Geometry check sheet. Reference: the model listing, model coordinates, mm. A direction names the side the tool comes from. Give positions to 0.01 mm unless a question says otherwise; leave off trailing zeros. Loops run counter-clockwise (first coordinate to the right, second up) from the corner with the lowest first, then second, coordinate; pieces in that order, holes last.
```python
from build123d import *

# Parameters (mm, degrees)
SKETCH1_R           = 60.5
SKETCH1_R_2         = 2.5
BOSS_EXTRUDE1_DEPTH = 5
SKETCH2_R           = 5
CUT_EXTRUDE1_DEPTH  = 2
SKETCH4_R           = 2
CUT_EXTRUDE2_DEPTH  = 86.612499087


with BuildPart() as part:
    # Sketch1 → Boss-Extrude1 (new body)
    with BuildSketch(Plane(origin=(0, 0, 0), x_dir=(1, 0, 0), z_dir=(0, 1, 0))):
        with Locations(Location((0, 0, 0), (0, 0, 270))):
            Circle(SKETCH1_R)
        with Locations(Location((0, 0, 0), (0, 0, 270))):
            Circle(SKETCH1_R_2, mode=Mode.SUBTRACT)
    extrude(amount=BOSS_EXTRUDE1_DEPTH)

    # Sketch2 → Cut-Extrude1 (cut)
    with BuildSketch(Plane.XZ):
        with Locations(Location((0, 53, 0), (0, 0, 270))):
            Circle(SKETCH2_R)
        with Locations(Location((53, 0, 0), (0, 0, 270))):
            Circle(SKETCH2_R)
        with Locations(Location((0, -53, 0), (0, 0, 270))):
            Circle(SKETCH2_R)
        with Locations(Location((-53, 0, 0), (0, 0, 270))):
            Circle(SKETCH2_R)
    extrude(amount=-CUT_EXTRUDE1_DEPTH, mode=Mode.SUBTRACT)

    # Sketch4 → Cut-Extrude2 (cut, through all)
    with BuildSketch(Plane(origin=(0, 2, 0), x_dir=(-1, 0, 0), z_dir=(0, -1, 0))):
        with Locations(Location((0, -53, 0), (0, 0, 90))):
            Circle(SKETCH4_R)
        with Locations(Location((-53, 0, 0), (0, 0, 90))):
            Circle(SKETCH4_R)
        with Locations(Location((0, 53, 0), (0, 0, 90))):
            Circle(SKETCH4_R)
        with Locations(Location((53, 0, 0), (0, 0, 90))):
            Circle(SKETCH4_R)
    extrude(amount=-CUT_EXTRUDE2_DEPTH, mode=Mode.SUBTRACT)


solid = part.part
```
1) Sectioned sample at B-B on x = 0. Enter the section's corners in (y, z).
2) Sectioned sample at C-C on y = 0.9. Enter the section's corners in (x, z), plus the area to 3 significant figures.
3) Sectioned sample at A-A on z = 0. Enter the section's corners in (x, y).
4) Tool access check on faces 4 (the cylindrical face through (0, 3, 55)), 5 (the flat face through (0.1, 2, -55.2)). Record the directions out of +Z, -Z, +X, -X, +Y, -Y that give a thin tool (end or side, any length) a straight path to the whole face; none if there is none.
5) Depth check by flat-ended pin: P1, Ø4.5, axis at x = -53, z = 0, coming from the -Y side; P2, Ø2, axis at x = 41.5, y = 1, coming from the -Z side; P3, Ø3, axis at x = 0, z = 0, coming from the -Y side; P4, Ø3, axis at x = -10.5, y = 4, coming from the -Z side. Enter the tip coordinate at first touch or a pass-through.
6) Scan lines: line 1 along X through (y, z) = (3.65, 0); line 2 along X through (y, z) = (0.95, 53); line 3 along X through (y, z) = (0.55, -54.5). Record each from-to range of solid material in increasing order.
7) Sectioned sample at D-D on z = 53. Enter the section's corners in (x, y).
8) Mould release check, pull along X, two halves, no side actions. Record for faces 1 (the flat face through (0.1, 2, 50.8)), 2 (the cylindrical face through (-59.06, 2.46, -13.12)), 3 (the flat face through (1, 5, 13)): +X half, -X half, draft (parallel to the pull), parting line (faces both ways), or undercut.
Determined:
1. outline: (0, -60.5) - (5, -60.5) - (5, -55) - (2, -55) - (2, -58) - (0, -58) - close; (0, -48) - (2, -48) - (2, -51) - (5, -51) - (5, -2.5) - (0, -2.5) - close; (0, 2.5) - (5, 2.5) - (5, 51) - (2, 51) - (2, 48) - (0, 48) - close; (0, 58) - (2, 58) - (2, 55) - (5, 55) - (5, 60.5) - (0, 60.5) - close
2. outline: circle Ø121 at (0, 0); hole circle Ø10 at (-53, 0); hole circle Ø10 at (0, -53); hole circle Ø10 at (0, 53); hole circle Ø5 at (0, 0); hole circle Ø10 at (53, 0)
2. area: 11,200 mm2
3. outline: (-60.5, 0) - (-58, 0) - (-58, 2) - (-55, 2) - (-55, 5) - (-60.5, 5) - close; (-51, 2) - (-48, 2) - (-48, 0) - (-2.5, 0) - (-2.5, 5) - (-51, 5) - close; (2.5, 0) - (48, 0) - (48, 2) - (51, 2) - (51, 5) - (2.5, 5) - close; (55, 2) - (58, 2) - (58, 0) - (60.5, 0) - (60.5, 5) - (55, 5) - close
4. face 4: +Y, -Y
4. face 5: -Y
5. P1: stops at y = 2
5. P2: stops at z = -44.94
5. P3: passes through
5. P4: stops at z = -59.83
6. line 1: x = -60.5 to -55, -51 to -2.5, 2.5 to 51, 55 to 60.5
6. line 2: x = -29.18 to -5, 5 to 29.18
6. line 3: x = -26.27 to -4.77, 4.77 to 26.27
7. outline: (-29.18, 0) - (-5, 0) - (-5, 2) - (-2, 2) - (-2, 5) - (-29.18, 5) - close; (2, 2) - (5, 2) - (5, 0) - (29.18, 0) - (29.18, 5) - (2, 5) - close
8. face 1: undercut
8. face 2: parting line
8. face 3: draft
